Input: dimensioned drawing with shaded views. Units: mm. Origin: part minimum x, y, z. Round coordinates to 2 decimals unless told otherwise and drop trailing zeros. Loops run counter-clockwise (first coordinate to the right, second up) from the corner with the lowest first, then second, coordinate; pieces in that order, holes last. Notation, with made-up numbers: (80.5, 49.25) - (133.5, 49.25) arc R25 cw to (133.5, 73.25) - close; hole circle Ø7 at (30.5, 52.5). An arc over 180 degrees is marked (long way). One line per question, with ' | ' between items. Start each with the question number.
1. Mould query, pull axis Z, two halves, no side actions, for the marked faces 1, 2 and 3. Classes: pulls with the +Z half, pulls with the -Z half, needs draft (parallel to the pull), parting line crosses it, or undercut.
2. Cut plane C-C (z = 21.5). Return loops of the section in (x, y).
3. Cut plane D-D (x = 27). Return loops of the section in (y, z) (1 decimal).
4. Ray query, line 1 (Z direction, x = 22, y = 2.5); line 2 (Z direction, x = 18.5, y = 0.65); line 3 (X direction, y = 2.85, z = 14). Return the intervals inside material, ascending.
5. Pin query (flat end, axial travel): pin 1 (1 mm diameter, centred on x = 31.5, y = 1, fed in from -Z); pin 2 (0.9 mm diameter, centred on x = 28.5, y = 1.5, fed in from -Z). Return the tip coordinate at first contact, or that it passes through.
6. Cut plane A-A (x = 32). Return loops of the section in (y, z).
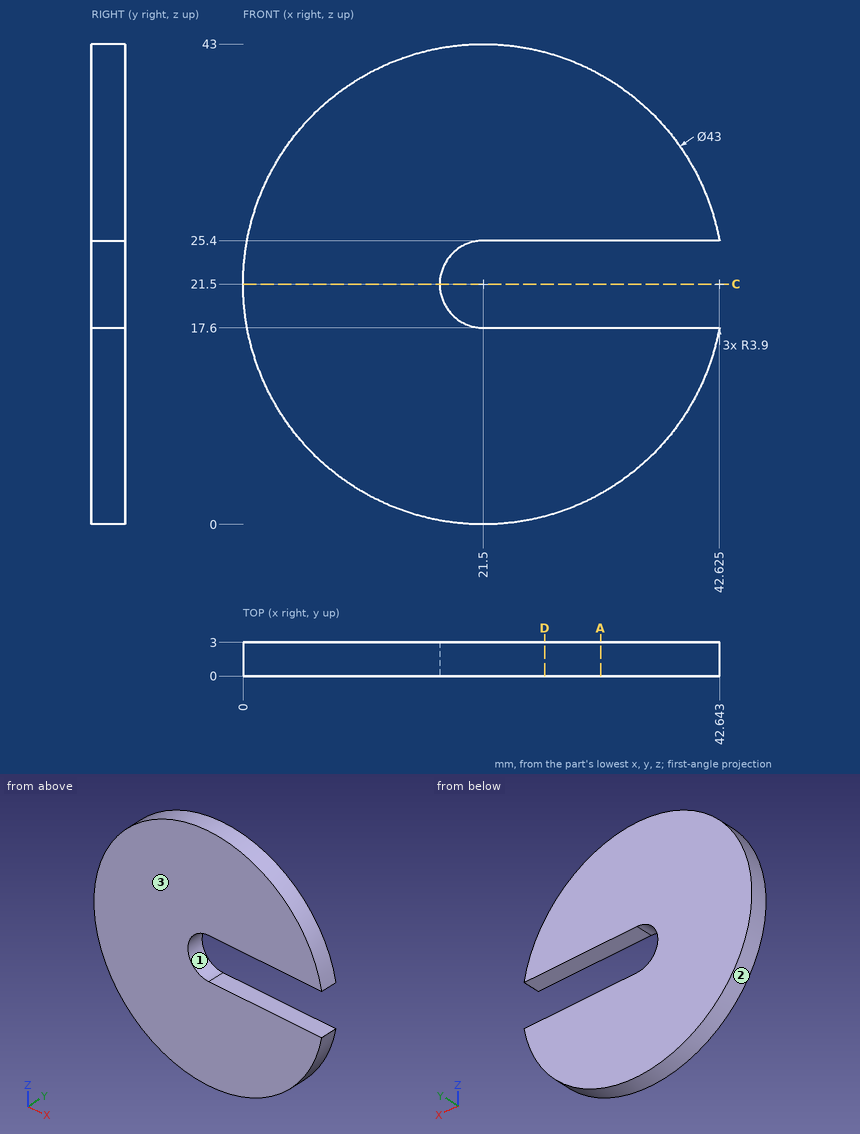
Answers follow:
1) face 1: undercut | face 2: parting line crosses it | face 3: needs draft
2) outline: (0, 0) - (17.6, 0) - (17.6, 3) - (0, 3) - close
3) outline: (0, 0.7) - (3, 0.7) - (3, 17.6) - (0, 17.6) - close; (0, 25.4) - (3, 25.4) - (3, 42.3) - (0, 42.3) - close
4) line 1: z = 0.01 to 17.6, 25.4 to 42.99 | line 2: z = 0.21 to 19.01, 23.99 to 42.79 | line 3: x = 1.35 to 41.65
5) pin 1: stops at z = 2.21 | pin 2: stops at z = 1.02
6) outline: (0, 2.74) - (3, 2.74) - (3, 17.6) - (0, 17.6) - close; (0, 25.4) - (3, 25.4) - (3, 40.26) - (0, 40.26) - close
